Can you work these out from the model? Positions are in its coordinate system, mm. A direction names the side the tool comes from. Coordinates: 2 decimals unless noted, no trailing zeros. Loops run counter-clockwise (first coordinate to the right, second up) from the corner with the lowest first, then second, coordinate; pieces in that order, holes last. Notation, with made-up numbers: (61.5, 68.25) -> (72.5, 68.25) arc R12 ccw to (72.5, 88.25) -> close; hole circle Ø5 at (80.25, 7.25). An arc over 180 degrees is marked (long way). Use one line per item in the form item = value. Start each with the question number.
(1) Imagine slicing it at B-B (z = 15). List the corners of the cut face in (x, y) for me, plus the area to 3 significant figures.
(2) On a 3-axis mill with a long thin cutter (end or side, diameter ignored), from which of +Z, -Z, +X, -X, +Y, -Y can I reach the whole of each face in a straight line? I mean faces 1 (the flat face through (-4, 23, 0)), 2 (the flat face through (-4, 23, 2)). Say none if no direction works.
(3) I need wall thicknesses on line 1 (Z direction, x = -44, y = 10); line 2 (Y direction, x = 159, z = 3.75). Which ranges of each line are inside material? Lowest first, please. Write a range as [from, to].
(4) Imagine slicing it at C-C (y = 32). List the corners of the cut face in (x, z) for me, plus the area to 3 significant figures.
(5) Imagine slicing it at A-A (x = -75). List the corners of the cut face in (y, z) for me.
(6) I'm going to push flat-ended pins straight in: pin 1 (5 mm diameter, centred on x = -161, y = 8, fed in from +Z); pin 2 (1.5 mm diameter, centred on y = 4.5, z = 16.5, fed in from -X); pin 3 (1 mm diameter, centred on x = -24.5, z = 8.5, fed in from +Y); pin 4 (12 mm diameter, centred on y = 28.5, z = 7.5, fed in from +X). Where does each tip first touch, or does it pass through?
Autodesk Inventor part; units mm, degrees
ref_plane "YZ Plane" through (0, 0, 0) normal (1, 0, 0) x (0, 1, 0)
ref_plane "XZ Plane" through (0, 0, 0) normal (0, 1, 0) x (-1, 0, 0)
ref_plane "XY Plane" through (0, 0, 0) normal (0, 0, 1) x (1, 0, 0)
sketch "Sketch1" plane through (0, 0, 0) normal (0, 0, 1) x (1, 0, 0)
  line L0 (-312.5, 40) -> (312.5, 40)
  line L1 (312.5, 40) -> (312.5, 0)
  line L2 (312.5, 0) -> (-312.5, 0)
  line L3 (-312.5, 0) -> (-312.5, 40)
  point P0 (0, 0)
  point P1 (0, 0)
  dimension "d1" = 40
  dimension "d45" = 625
extrude "Plate1" add sketch "Sketch1" along normal blind 2
sketch "Sketch2" plane through (312.5, 2, 0) normal (0, -1, 0) x (1, 0, 0)
  line L0 (-625, 0) -> (0, 0)
  line L1 (0, 0) -> (0, 20)
  line L2 (0, 20) -> (-625, 20)
  line L3 (-625, 20) -> (-625, 0)
edge flange "Flange1" height 20 angle 90 thickness 2 bend radius 2.75 thickness toward (0, -1, 0) relief round relief width 2 relief depth 1 edges at (0, 0, 2) wall of the first edge with corners at (-312.5, 2, 0) (312.5, 2, 0) (312.5, 2, 20) (-312.5, 2, 20)
bend "Bend1"
corner "Corner1"
sketch "Sketch6" plane through (0, 0, 0) normal (0, 0, -1) x (-1, 0, 0)
  line L0 (-312.5, 40) -> (-312.5, 4.75)
  circle A0 centre (-312.5, 40) radius 22.5
  line L1 (-312.5, 40) -> (312.5, 40)
  line L2 (-499, 30) -> (-499, 67.6691)
  point P0 (0, 0)
  point P1 (-290, 40)
  point P2 (-312.5, 17.5)
  point P3 (312.5, 40)
  dimension "d24" = 45
extrude "Extrusion2" cut sketch "Sketch6" along normal mid plane 30 contours L1 A0 L0 picked at (-297.688, 38.3311)
sketch "Sketch9" plane through (0, 0, 2) normal (0, 0, 1) x (1, 0, 0)
  line L0 (95.482, 35) -> (95.482, 23) construction
  line L1 (95.482, 23) -> (-104.518, 23) construction
  line L2 (-104.518, 23) -> (-104.518, 35) construction
  line L3 (-104.518, 35) -> (95.482, 35) construction
  line L4 (-312.5, 40) -> (312.5, 40)
  point P0 (0, 0)
  dimension "d40" = 200
  dimension "d41" = 12
  dimension "d43" = 5
mark "Mark2"
mirror "Mirror3" about plane through (0, 0, 0) normal (1, 0, 0) of "Extrusion2"
equation "\"d43\" = d42"
equation "\"d2\" = Thickness"
equation "\"d3\" = BendReliefWidth"
equation "\"d4\" = BendReliefDepth"
equation "\"d5\" = MinimumRemnant"
equation "\"d6\" = TransitionRadius"
equation "\"d9\" = BendRadius"
equation "\"d10\" = CornerReliefSize"
equation "\"d11\" = GapSize"
equation "\"d12\" = JacobiRadiusSize"
equation "\"GapSize\" = Thickness"
equation "\"MinimumRemnant\" = 2 * Thickness"
equation "\"BendReliefDepth\" = 0.5 * Thickness"
equation "\"BendReliefWidth\" = Thickness"
equation "\"CornerReliefSize\" = 4 * Thickness"
equation "\"JacobiRadiusSize\" = BendRadius"
equation "\"TransitionRadius\" = BendRadius"
equation "\"qqqqqq\" = 67.35706"
properties part number "MSC 408 STRINGER LOWERBACK" material "Stainless Steel"
Worked out:
q1.outline = (-312.5, 0) -> (312.5, 0) -> (312.5, 2) -> (-312.5, 2) -> close
q1.area = 1,250 mm2
q2.face_1 = -Z, +X, -X, +Y, -Y
q2.face_2 = +Z, +X, -X, +Y
q3.line_1 = [0, 2]
q3.line_2 = [0.11, 2.19]
q4.outline = (-291.47, 0) -> (291.47, 0) -> (291.47, 2) -> (-291.47, 2) -> close
q4.area = 1,170 mm2
q5.outline = (0, 4.75) arc R4.75 ccw to (4.75, 0) -> (40, 0) -> (40, 2) -> (4.75, 2) arc R2.75 cw to (2, 4.75) -> (2, 20) -> (0, 20) -> close
q6.pin_1 = 2
q6.pin_2 = through
q6.pin_3 = 2
q6.pin_4 = 294.81
